from build123d import *

# Parameters (mm, degrees)
SKETCH_18_W            = 200
SKETCH_18_H            = 100
SM_BASE_FLANGE_3_DEPTH = 1.5
SKETCH_23_W            = 55
SKETCH_23_H            = 15
SKETCH_23_W_2          = 47.5
SKETCH_23_H_2          = 20
CUT_EXTRUDE_1_DEPTH    = 1.5
CUT_EXTRUDE_2_DEPTH    = 1.5
OTHER_START            = -52.5
OTHER_2_DEPTH          = 105
OTHER_2_2_DEPTH        = 105
FILLET_1_R             = 4
SKETCH_26_R            = 2.1
CUT_EXTRUDE_3_DEPTH    = 1.5


# Read off the part's stored shape, not the designer's step: 绘制的折弯2
# Sheet-metal steps are written as plain solids
with BuildPart() as part:
    # 草图18 → 基体-法兰3 (new body)
    with BuildSketch(Plane(origin=(0, 0, 0), x_dir=(1, 0, 0), z_dir=(0, 1, 0))):
        Rectangle(SKETCH_18_W, SKETCH_18_H)
    extrude(amount=-SM_BASE_FLANGE_3_DEPTH)

    # 草图23 → 切除-拉伸1 (cut)
    with BuildSketch(Plane(origin=(0, 0, 0), x_dir=(1, 0, 0), z_dir=(0, 1, 0))):
        with Locations((27.5, 42.5)):
            Rectangle(SKETCH_23_W, SKETCH_23_H)
        with Locations((-27.5, 42.5)):
            Rectangle(SKETCH_23_W, SKETCH_23_H)
        with Locations((76.25, -40)):
            Rectangle(SKETCH_23_W_2, SKETCH_23_H_2)
        with Locations((-76.25, -40)):
            Rectangle(SKETCH_23_W_2, SKETCH_23_H_2)
    extrude(amount=-CUT_EXTRUDE_1_DEPTH, mode=Mode.SUBTRACT)

    # 草图24 → 切除-拉伸2 (cut)
    with BuildSketch(Plane(origin=(0, 0, 0), x_dir=(1, 0, 0), z_dir=(0, 1, 0))):
        Polygon((-52.5, -30), (-55, -5), (-67.872428489, -30), align=None)
        Polygon((55, -5), (67.872428489, -30), (52.5, -30), align=None)
    extrude(amount=-CUT_EXTRUDE_2_DEPTH, mode=Mode.SUBTRACT)

    # Other 2 outline → Other 2 (cut)
    with BuildSketch(Plane.YZ.offset(OTHER_START)):
        with BuildLine():
            ThreePointArc((-1.5, 30), (-1.086838938, 31.295164082), (0, 32.111823856))
            Line((0, 32.111823856), (0, 50))
            Line((0, 50), (-1.5, 50))
            Line((-1.5, 50), (-1.5, 30))
        make_face()
    extrude(amount=OTHER_2_DEPTH, mode=Mode.SUBTRACT)

    # Other 2 2 outline → Other 2 2 (add)
    with BuildSketch(Plane.YZ.offset(OTHER_START)):
        with BuildLine():
            Line((18.401454181, 30.7366), (18.401454181, 32.2366))
            Line((18.401454181, 32.2366), (0.7366, 32.2366))
            ThreePointArc((0.7366, 32.2366), (0.363053267, 32.205185343), (0, 32.111823856))
            Line((0, 32.111823856), (0, 30))
            ThreePointArc((0, 30), (0.215745145, 30.520854855), (0.7366, 30.7366))
            Line((0.7366, 30.7366), (18.401454181, 30.7366))
        make_face()
    extrude(amount=OTHER_2_2_DEPTH)

    # 圆角1
    fillet_1_edges = [part.edges().sort_by_distance(p)[0] for p in [
        (67.872428489, -0.75, 30),
        (100, -0.75, 30),
        (100, -0.75, -50),
        (55, -0.75, -50),
        (55, -0.75, -35),
        (-55, -0.75, -35),
        (-55, -0.75, -50),
        (-100, -0.75, -50),
        (-100, -0.75, 30),
        (-67.872428489, -0.75, 30),
        (52.5, 18.401454181, 31.4866),
        (-52.5, 18.401454181, 31.4866),
    ]]
    fillet(fillet_1_edges, radius=FILLET_1_R)

    # 草图26 → 切除-拉伸3 (cut)
    with BuildSketch(Plane(origin=(0, 0, 0), x_dir=(1, 0, 0), z_dir=(0, 1, 0))):
        with Locations(Location((-96, 46, 0), (0, 0, 270))):
            Circle(SKETCH_26_R)
        with Locations(Location((-96, 33.3, 0), (0, 0, 270))):
            Circle(SKETCH_26_R)
        with Locations(Location((96, 33.3, 0), (0, 0, 90))):
            Circle(SKETCH_26_R)
        with Locations(Location((96, 46, 0), (0, 0, 90))):
            Circle(SKETCH_26_R)
    extrude(amount=-CUT_EXTRUDE_3_DEPTH, mode=Mode.SUBTRACT)


solid = part.part
Could you check a few things on this model? Use its own coordinates, in mm. A direction names the side the tool comes from. Round coordinates to 2 decimals unless told otherwise and drop trailing zeros. Order: outer loops, then holes, each group sorted by start corner. A loop starts at its lowest first (then second) coordinate and runs counter-clockwise, first axis right, second up. Notation, with made-up numbers: M 32.25,87 L 90.25,87 A26 cw 90.25,113 Z; hole C 45,20 d11. An arc over 180 degrees is marked long. One line per item, written item: value.
(1) Imagine slicing it at B-B (x = 17). Write out the boundary of the cut face in (y, z), and give its area (4 significant figures).
Ans:
outline: M -1.5,-35 L 0,-35 L 0,30 A0.74 cw 0.74,30.74 L 18.4,30.74 L 18.4,32.24 L 0.74,32.24 A2.24 ccw -1.5,30 Z
area: 127.5 mm^2
(2) Which directions (+Z, -Z, +X, -X, +Y, -Y) give clear straight access to the entire face, cutting with the end or side of a thin tool? Please do faces 5 (the cylindrical face through (98.797, -0.76, -48.859)), 6 (the cylindrical face through (98.859, -0.76, 28.797)), 7 (the cylindrical face through (-56.203, -0.76, -48.859)), 8 (the flat face through (-1, 9, 30.737)), 9 (the flat face through (-60.796, -0.74, 16.256)).
Ans:
face 5: -Z, +X, +Y, -Y
face 6: +Z, +X, +Y, -Y
face 7: -Z, +Y, -Y
face 8: -Z, +X, -X, +Y
face 9: +Z, +Y, -Y
(3) I'm going to push flat-ended pins straight in: P1, Ø2.5, axis at y = 7.5, z = 31, coming from the +X side; P2, Ø3.5, axis at x = -96, z = -46, coming from the -Y side; P3, Ø3, axis at x = -65.5, z = -7.5, coming from the +Y side; P4, Ø6.5, axis at x = -96, z = -33.3, coming from the -Y side. Where does each tip first touch, or does it pass through?
Ans:
P1: stops at x = 52.5
P2: passes through
P3: stops at y = 0
P4: stops at y = -1.5
(4) Imagine slicing it at A-A (z = -33). Write out the boundary of the cut face in (x, y).
Ans:
outline: M -100,-1.5 L -98.08,-1.5 L -98.08,0 L -100,0 Z; M -93.92,-1.5 L 93.92,-1.5 L 93.92,0 L -93.92,0 Z; M 98.08,-1.5 L 100,-1.5 L 100,0 L 98.08,0 Z
(5) Imagine slicing it at D-D (z = -23.5). Write out the boundary of the cut face in (x, y), and give its area (3 significant figures).
Ans:
outline: M -100,-1.5 L 100,-1.5 L 100,0 L -100,0 Z
area: 300 mm^2
(6) Imagine slicing it at C-C (y = 12.25). Write out the boundary of the cut face in (x, z).
Ans:
outline: M -52.5,30.74 L 52.5,30.74 L 52.5,32.24 L -52.5,32.24 Z
(7) I need wall thicknesses on line 1 along X through (y, z) = (-0.45, -33.3); line 2 along Z through (x, y) = (96, -0.9); line 3 along X through (y, z) = (-0.35, -46). Which ranges of each line are inside material? Lowest first, please. Write a range as from..to.
Ans:
line 1: x = -100..-98.1, -93.9..93.9, 98.1..100
line 2: z = -50..-48.1, -43.9..-35.4, -31.2..30
line 3: x = -100..-98.1, -93.9..-55, 55..93.9, 98.1..100
(8) If we mould it in two halves opening along Z, with no side actions, what happens to faces 1 (the cylindrical face through (97.278, -0.74, -31.634)), 2 (the cylindrical face through (51.3, 17.26, 31.5)), 3 (the cylindrical face through (-98.859, -0.76, 28.797)), 4 (the cylindrical face through (-53.859, -0.76, -36.203))? For each: released by +Z, released by -Z, zero draft, split by the parting line, or undercut.
Ans:
face 1: undercut
face 2: zero draft
face 3: released by +Z
face 4: released by -Z
